Work out the finished part from the listing and answer in its coordinate system (mm). Face numbers are marked on the shaded views. A direction names the side the tool comes from. Round coordinates to 2 decimals unless told otherwise and drop trailing zeros. Write each loop counter-clockwise with the first axis right and the second up, starting at its lowest first coordinate (ties: lowest second). Pieces come first, ordered by that corner, then holes. Notation, with made-up numbers: M 79,86.5 L 95,86.5 A31 cw 95,121.5 Z; hole C 73,40 d8. An arc over 180 degrees is marked long. Answer in a Markdown table with one row per item.
```python
from build123d import *

# Parameters (mm, degrees)
SKETCH1_W           = 70
SKETCH1_H           = 110
BOSS_EXTRUDE1_DEPTH = 3
SKETCH2_W           = 70
SKETCH2_H           = 3
BOSS_EXTRUDE2_DEPTH = 50
SKETCH3_R           = 2
CUT_EXTRUDE1_DEPTH  = 3


with BuildPart() as part:
    # Sketch1 → Boss-Extrude1 (new body)
    with BuildSketch(Plane.XY):
        Rectangle(SKETCH1_W, SKETCH1_H)
    extrude(amount=BOSS_EXTRUDE1_DEPTH)

    # Sketch2 → Boss-Extrude2 (add)
    with BuildSketch(Plane(origin=(0, 0, 0), x_dir=(-1, 0, 0), z_dir=(0, 0, -1))):
        with Locations((0, -53.5)):
            Rectangle(SKETCH2_W, SKETCH2_H)
    extrude(amount=BOSS_EXTRUDE2_DEPTH)

    # Sketch3 → Cut-Extrude1 (cut)
    with BuildSketch(Plane.XY.offset(3)):
        with Locations((-28.5, 50)):
            Circle(SKETCH3_R)
        with Locations((28.5, 50)):
            Circle(SKETCH3_R)
    extrude(amount=-CUT_EXTRUDE1_DEPTH, mode=Mode.SUBTRACT)


solid = part.part
```
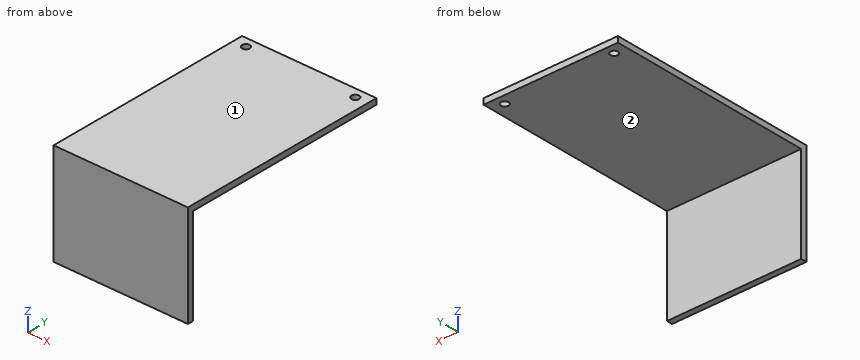
1. The part is cut by section C-C (z = -14.5). Determine the outline of the cut face in (x, y), plus the area to 3 significant figures.
Calculated:
| item | result |
|---|---|
| outline | M -35,-55 L 35,-55 L 35,-52 L -35,-52 Z |
| area | 210 mm² |
2. The part is cut by section A-A (x = -28.5). Determine the outline of the cut face in (y, z).
Calculated:
| item | result |
|---|---|
| outline | M -55,-50 L -52,-50 L -52,0 L 48,0 L 48,3 L -55,3 Z; M 52,0 L 55,0 L 55,3 L 52,3 Z |
3. A tool of negligible diameter and unlimited length cuts with its end or side. For the marked faces 1 and 2, from which of +Z, -Z, +X, -X, +Y, -Y can it reach the whole face along a straight path? Write none if from no direction.
Calculated:
| item | result |
|---|---|
| face 1 | +Z, +X, -X, +Y, -Y |
| face 2 | -Z, +X, -X, +Y |
4. Given pin 1 (3 mm diameter, centred on x = 28.5, y = 50, fed in from -Z); pin 2 (4 mm diameter, centred on x = -4, y = 8.5, fed in from -Z), each flat-ended and moving along its own axis, determine where each tip first touches the part or whether it passes through.
Calculated:
| item | result |
|---|---|
| pin 1 | passes through |
| pin 2 | stops at z = 0 |
5. The part is cut by section B-B (y = 50). Determine the outline of the cut face in (x, z).
Calculated:
| item | result |
|---|---|
| outline | M -35,0 L -30.5,0 L -30.5,3 L -35,3 Z; M -26.5,0 L 26.5,0 L 26.5,3 L -26.5,3 Z; M 30.5,0 L 35,0 L 35,3 L 30.5,3 Z |
6. Consider line 1 along Y through (x, z) = (-28.5, 0.95); line 2 along Y through (x, z) = (-7, -37.5); line 3 along Z through (x, y) = (-11.5, 16). Determine where each line is inside the solid, lowest interval first. Write a range as from..to.
Calculated:
| item | result |
|---|---|
| line 1 | y = -55..48, 52..55 |
| line 2 | y = -55..-52 |
| line 3 | z = 0..3 |
7. The part is cut by section D-D (x = 11.5). Determine the outline of the cut face in (y, z).
Calculated:
| item | result |
|---|---|
| outline | M -55,-50 L -52,-50 L -52,0 L 55,0 L 55,3 L -55,3 Z |
